Read the model definition and answer for the solid it produces. Units are mm, in the model's axes. A direction names the side the tool comes from. Give positions to 0.01 mm unless a question says otherwise; leave off trailing zeros. Order: outer loops, then holes, each group sorted by start corner. A loop starts at its lowest first (then second) coordinate and runs counter-clockwise, first axis right, second up. Notation, with made-up numbers: (17, -31) - (60, -31) arc R24 ccw to (60, -6) - close; hole circle Ø1 at (55.5, 38.25). An arc over 180 degrees is marked (long way). Write each question's results on one line, items separated by ' | '. Start each with the question number.
Q1. Flat-ended cylindrical pins translate along their axes: P1, Ø5.5, axis at y = 8.5, z = 3, coming from the +X side; P2, Ø3.5, axis at x = -8, z = 7, coming from the +Y side; P3, Ø3, axis at x = -10.5, y = 1, coming from the +Z side. Find the tip coordinate at first contact, or state that the pin passes through.
Q2. A tool of negligible diameter and unlimited length cuts with its end or side. For faces 4 (the face through (-1, 8, 1.5)), 5 (the face through (4.54, 8, 4)), 6 (the face through (1.035, 14.466, 1.824)), from which of +Z, -Z, +X, -X, +Y, -Y can it reach the whole face along a straight path? Write none if from no direction.
Q3. Find section B-B on y = 0. Give the vertices of the cut face in (x, z).
Q4. Find section D-D on z = 13. Give the vertices of the cut face in (x, y).
Q5. Find the intervals of material crossed by line 1 along X through (y, z) = (9.5, 7.25); line 2 along Y through (x, z) = (-9.5, 0.9); line 3 along Y through (x, z) = (-7.5, 6.25), in increasing order. Write a range as from..to.
Q6. For a pull along X with two mould halves and no side action, classify faces 1 (the face through (-1.007, 14.465, 1.824)), 2 (the face through (-5.386, 4.337, 6.117)), 3 (the face through (4.71, 1.48, 14.28)) as +X half, -X half, draft (parallel to the pull), parting line (faces both ways), or undercut.
Q7. Find section C-C on z = 6.5. Give the vertices of the cut face in (x, y).
Q8. Find section A-A on z = 3. Give the vertices of the cut face in (x, y).
from build123d import *

# Parameters (mm, degrees)
SKETCH_R     = 3
PAD_DEPTH    = 15
SKETCH002_R  = 1.5
PAD001_DEPTH = 1.5


with BuildPart() as part:
    # Sketch → Pad (new body)
    with BuildSketch(Plane.XY):
        Polygon((0, 14.427438), (-2.041881, 14.502734), (-4.540238, 12.582665), (-4.540238, 8.140154), (-4.540238, 5.954917), (-4.912402, 4.43243), (-5.873682, 4.237903), (-12.981692, 4.237903), (-14.428203, 1.815223), (-14.428203, 0), (-14.428203, -2.157977), (-13.184835, -4.115694), (-6.069288, -4.115694), (-3.269161, -8.313478), (0, -8.313478), (3.269161, -8.313478), (6.069288, -4.115694), (13.184835, -4.115694), (14.428203, -2.157977), (14.428203, 0), (14.428203, 1.815223), (12.981692, 4.237903), (5.873682, 4.237903), (4.912402, 4.43243), (4.540238, 5.954917), (4.540238, 8.140154), (4.540238, 12.582665), (2.041881, 14.502734), align=None)
        with Locations((0, 9.5)):
            Circle(SKETCH_R, mode=Mode.SUBTRACT)
        with Locations((-9.5, 0)):
            Circle(SKETCH_R, mode=Mode.SUBTRACT)
        with Locations((9.5, 0)):
            Circle(SKETCH_R, mode=Mode.SUBTRACT)
    extrude(amount=PAD_DEPTH)

    # Sketch001 → Groove (revolve, cut)
    with BuildSketch(Plane.XZ):
        Polygon((3.000144, 16.438543), (15.461766, 2.546283), (18.059507, 16.438543), align=None)
    revolve(axis=Axis((0, 0, 0), (0, 0, 1)), mode=Mode.SUBTRACT)

    # Sketch002 (on Face2 of Groove) → Pad001 (join)
    with BuildSketch(Plane(origin=(0, 0, 0), x_dir=(1, 0, 0), z_dir=(0, 0, -1))):
        Polygon((-12.307145, 3.302316), (11.637245, 3.302316), (13.331424, 0.817521), (13.067885, -2.119055), (11.185462, -3.474398), (3.392242, -3.474398), (3.655782, -9.272253), (2.940462, -12.66061), (0.342722, -13.37593), (-2.895042, -12.773556), (-3.873901, -9.159308), (-3.459768, -4.528554), (-5.455134, -2.984969), (-11.70477, -3.737936), (-13.737784, -1.366087), align=None)
        with Locations((-9.5, 0)):
            Circle(SKETCH002_R, mode=Mode.SUBTRACT)
        with Locations((9.5, 0)):
            Circle(SKETCH002_R, mode=Mode.SUBTRACT)
        with Locations((0, -9.5)):
            Circle(SKETCH002_R, mode=Mode.SUBTRACT)
    extrude(amount=-PAD001_DEPTH)


solid = part.part
Working result:
1) P1: x = 4.59 | P2: y = 4.24 | P3: z = 1.5
2) face 4: +Z | face 5: +Z, -Z, +X, +Y | face 6: +Z, -Z, +Y
3) outline: (-14.43, 0) - (-11, 0) - (-11, 1.5) - (-12.5, 1.5) - (-12.5, 5.85) - (-14.43, 3.7) - close; (-8, 0) - (8, 0) - (8, 1.5) - (6.5, 1.5) - (6.5, 12.54) - (4.29, 15) - (-4.29, 15) - (-6.5, 12.54) - (-6.5, 1.5) - (-8, 1.5) - close; (11, 0) - (14.43, 0) - (14.43, 3.7) - (12.5, 5.85) - (12.5, 1.5) - (11, 1.5) - close
4) outline: circle Ø12.17 at (0, 0)
5) line 1: -4.54..-3, 3..4.54 | line 2: -4.12..-1.5, 1.5..4.24 | line 3: -4.12..-2.24, 2.24..4.24
6) face 1: undercut | face 2: -X half | face 3: parting line
7) outline: (-11.75, -1.99) arc R11.92 ccw to (-11.18, -4.12) - (-6.07, -4.12) - (-3.27, -8.31) - (3.27, -8.31) - (6.07, -4.12) - (11.18, -4.12) arc R11.92 ccw to (11.75, -1.99) arc R3 cw (long way) to (11.75, 1.99) arc R11.92 ccw to (11.14, 4.24) - (5.87, 4.24) - (4.91, 4.43) - (4.54, 5.95) - (4.54, 11.02) arc R11.92 ccw to (1.99, 11.75) arc R3 cw (long way) to (-1.99, 11.75) arc R11.92 ccw to (-4.54, 11.02) - (-4.54, 5.95) - (-4.91, 4.43) - (-5.87, 4.24) - (-11.14, 4.24) arc R11.92 ccw to (-11.75, 1.99) arc R3 cw (long way) to start
8) outline: (-14.43, -2.16) - (-13.18, -4.12) - (-6.07, -4.12) - (-3.27, -8.31) - (3.27, -8.31) - (6.07, -4.12) - (13.18, -4.12) - (14.43, -2.16) - (14.43, 1.82) - (12.98, 4.24) - (5.87, 4.24) - (4.91, 4.43) - (4.54, 5.95) - (4.54, 12.58) - (2.04, 14.5) - (0, 14.43) - (-2.04, 14.5) - (-4.54, 12.58) - (-4.54, 5.95) - (-4.91, 4.43) - (-5.87, 4.24) - (-12.98, 4.24) - (-14.43, 1.82) - close; hole circle Ø6 at (-9.5, 0); hole circle Ø6 at (0, 9.5); hole circle Ø6 at (9.5, 0)
